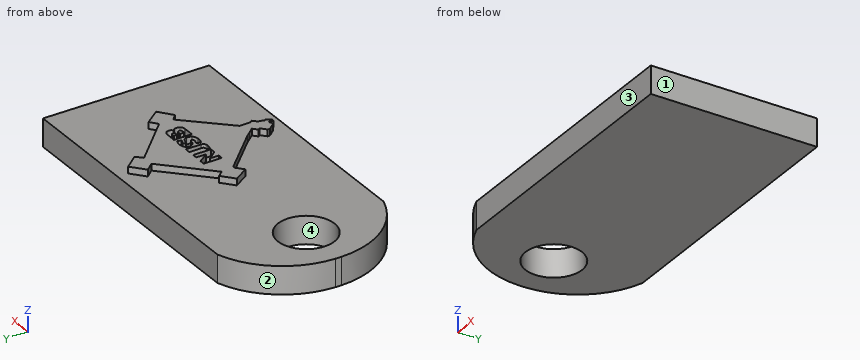
from build123d import *

# Parameters (mm, degrees)
F0_W     = 38.1
F0_H     = 19.05
F1_DEPTH = 3.175
F2_R     = 3.239621
F3_DEPTH = 3.176
F5_DEPTH = 0.762


with BuildPart() as f1:
    # F0 (on Top) → F1 (new body)
    with BuildSketch(Plane.XY):
        with Locations((-19.05, 9.525)):
            Rectangle(F0_W, F0_H)
    extrude(amount=F1_DEPTH)

    # F2 (on face) → F3 (cut, through all)
    with BuildSketch(Plane.XY.offset(3.175)):
        with BuildLine():
            ThreePointArc((-38.1, 9.877407), (-36.161286, 15.559844), (-31.275846, 19.05))
            Line((-31.275846, 19.05), (-38.1, 19.05))
            Line((-38.1, 19.05), (-38.1, 9.877407))
        make_face()
        with BuildLine():
            ThreePointArc((-31.275846, 0), (-36.161286, 3.490156), (-38.1, 9.172593))
            Line((-38.1, 9.172593), (-38.1, 0))
            Line((-38.1, 0), (-31.275846, 0))
        make_face()
        with Locations((-32.302372, 9.525)):
            Circle(F2_R)
    extrude(amount=-F3_DEPTH, mode=Mode.SUBTRACT)

    # F4 (on face) → F5 (join)
    with BuildSketch(Plane.XY.offset(3.175)):
        Polygon((-12.133155, 16.323839), (-13.419535, 17.867444), (-14.930828, 16.581235), (-14.155187, 15.669858), (-19.111004, 10.793301), (-19.653987, 11.431306), (-21.029584, 10.260583), (-19.947039, 8.606749), (-19.111004, 9.318269), (-18.885918, 9.318269), (-14.609277, 4.973212), (-14.512812, 5.356764), (-14.512812, 5.616316), (-14.239308, 6.20037), (-14.159105, 6.484506), (-12.678197, 6.066489), (-12.678197, 5.356764), (-12.937207, 5.101833), (-12.937207, 4.555195), (-12.549366, 4.555195), (-8.081773, 9.282008), (-7.436184, 8.671823), (-5.89522, 9.860801), (-7.199443, 11.551126), (-8.05396, 10.891797), (-12.808586, 15.648736), align=None)
        Polygon((-16.313503, 9.314163), (-16.86014, 9.346317), (-16.86014, 11.40425), (-16.281348, 11.40425), (-15.445312, 10.214509), (-15.445312, 11.372095), (-14.898674, 11.372095), (-14.898674, 9.314163), (-15.509622, 9.314163), (-16.313503, 10.310974), align=None, mode=Mode.SUBTRACT)
        with BuildLine():
            Line((-14.210255, 9.967692), (-14.223414, 11.372095))
            Line((-14.223414, 11.372095), (-13.580311, 11.372095))
            Line((-13.580311, 11.372095), (-13.580311, 9.642933))
            ThreePointArc((-13.580311, 9.642933), (-13.703139, 9.33071), (-14.005777, 9.185865))
            ThreePointArc((-14.005777, 9.185865), (-14.361345, 9.206839), (-14.703408, 9.306146))
            Line((-14.703408, 9.306146), (-14.595155, 9.691046))
            ThreePointArc((-14.595155, 9.691046), (-14.309597, 9.699827), (-14.210255, 9.967692))
        make_face(mode=Mode.SUBTRACT)
        with BuildLine():
            Line((-12.309813, 11.38701), (-11.792604, 11.230645))
            Line((-11.792604, 11.230645), (-11.919432, 10.779702))
            Line((-11.919432, 10.779702), (-12.419279, 10.920285))
            ThreePointArc((-12.419279, 10.920285), (-12.566064, 10.888649), (-12.622545, 10.74952))
            ThreePointArc((-12.622545, 10.74952), (-12.370625, 10.614414), (-12.093307, 10.545042))
            ThreePointArc((-12.093307, 10.545042), (-11.848866, 10.36705), (-11.732464, 10.087973))
            ThreePointArc((-11.732464, 10.087973), (-11.733256, 9.7951), (-11.840717, 9.522652))
            ThreePointArc((-11.840717, 9.522652), (-12.10655, 9.335291), (-12.419279, 9.246006))
            Line((-12.419279, 9.246006), (-12.827022, 9.246006))
            Line((-12.827022, 9.246006), (-13.272062, 9.390343))
            Line((-13.272062, 9.390343), (-13.113701, 9.878622))
            Line((-13.113701, 9.878622), (-12.726019, 9.752887))
            ThreePointArc((-12.726019, 9.752887), (-12.49708, 9.751795), (-12.309813, 9.883496))
            ThreePointArc((-12.309813, 9.883496), (-12.54216, 10.088347), (-12.851078, 10.111114))
            ThreePointArc((-12.851078, 10.111114), (-13.120867, 10.31145), (-13.28409, 10.605182))
            ThreePointArc((-13.28409, 10.605182), (-13.263213, 10.944513), (-13.079613, 11.230645))
            ThreePointArc((-13.079613, 11.230645), (-12.708492, 11.376665), (-12.309813, 11.38701))
        make_face(mode=Mode.SUBTRACT)
        with BuildLine():
            Line((-11.43176, 9.294118), (-11.43176, 11.350926))
            Line((-11.43176, 11.350926), (-10.087523, 11.330864))
            Line((-10.087523, 11.330864), (-9.940274, 11.266729))
            ThreePointArc((-9.940274, 11.266729), (-9.644752, 10.815674), (-9.940274, 10.36462))
            ThreePointArc((-9.940274, 10.36462), (-9.820796, 10.300702), (-9.711741, 10.220283))
            ThreePointArc((-9.711741, 10.220283), (-9.661743, 9.61308), (-10.180837, 9.294118))
            Line((-10.180837, 9.294118), (-11.43176, 9.294118))
        make_face(mode=Mode.SUBTRACT)
        with BuildLine():
            Line((-10.445168, 10.196227), (-10.770215, 10.208255))
            Line((-10.770215, 10.208255), (-10.770215, 9.751187))
            Line((-10.770215, 9.751187), (-10.445168, 9.746336))
            ThreePointArc((-10.445168, 9.746336), (-10.216841, 9.971281), (-10.445168, 10.196227))
        make_face()
        with BuildLine():
            Line((-10.770215, 10.929941), (-10.770215, 10.55707))
            Line((-10.770215, 10.55707), (-10.493567, 10.55707))
            ThreePointArc((-10.493567, 10.55707), (-10.307132, 10.743506), (-10.493567, 10.929941))
            Line((-10.493567, 10.929941), (-10.770215, 10.929941))
        make_face()
        Polygon((-12.549366, 3.912091), (-12.549366, 4.555195), (-12.937207, 4.555195), (-12.937207, 5.101833), (-12.678197, 5.356764), (-12.678197, 6.066489), (-14.159105, 6.484506), (-14.239308, 6.20037), (-14.512812, 5.616316), (-14.512812, 5.356764), (-14.609277, 4.973212), (-14.421192, 4.752211), (-14.170298, 4.457412), (-13.643861, 3.838849), (-14.170298, 3.390817), (-13.987954, 3.176562), (-14.609277, 2.647775), (-14.609277, 2.368642), (-14.346565, 2.059955), (-13.987954, 1.638587), (-13.643861, 1.638587), (-13.430775, 1.819937), (-13.430775, 1.24321), (-13.162293, 1.24321), (-12.872897, 1.819937), (-13.028217, 1.897875), (-12.827437, 2.298001), (-12.827437, 2.561572), (-12.326258, 3.0439), (-12.549366, 3.275728), align=None)
    extrude(amount=F5_DEPTH)


solid = f1.part
Can you work these out from the model? Positions are in its coordinate system, mm. Face numbers are marked on the shaded views. Give positions to 0.01 mm unless a question says otherwise; leave off trailing zeros. Write each loop counter-clockwise with the first axis right and the second up, starting at its lowest first coordinate (ties: lowest second). Pieces come first, ordered by that corner, then holes. Notation, with made-up numbers: M -10,-9.75 L 17,-9.75 A29 cw 17,17.25 Z; hole C -36.5,0 d6. An arc over 180 degrees is marked long. Answer in a Markdown table with one row per item. Add a question column.
Item 1: Imagine slicing it at C-C, the plane z = 2. Write out the boundary of the cut face in (x, y) (3 decimals).
Item 2: We'd pull the mould along X, two halves only. Please class the marked faces 1, 2, 3 and 4: released by +X, released by -X, zero draft, split by the parting line, or undercut.
Item 3: For pin 1 Ø1.2 at (x, y) = (-14, 10) entering from +Z, with a flat end and sliding along its axis, tell me the tip position at first contact or that it passes through.
Item 4: Imagine slicing it at D-D, the plane x = -18.5. Write out the boundary of the cut face in (y, z) (3 decimals), plus the area to 3 significant figures.
Item 5: Please list where these lines run through material, in increasing order: L1, parallel to Z at x = -29, y = 7 (3 decimals); L2, parallel to X at y = 9.5, z = 0.8; L3, parallel to Y at x = -31, z = 0.85.
Item 6: Imagine slicing it at B-B, the plane x = -32. Write out the boundary of the cut face in (y, z) (3 decimals), plus the area to 3 significant figures.
Item 7: Imagine slicing it at A-A, the plane y = 7.25. Write out the boundary of the cut face in (x, z) (3 decimals).
Evaluation:
| question | item | result |
|---|---|---|
| 1 | outline | M -38.1,9.173 A9.815 ccw -31.276,0 L 0,0 L 0,19.05 L -31.276,19.05 A9.815 ccw -38.1,9.877 Z; hole C -32.302,9.525 d6.479 |
| 2 | face 1 | released by +X |
| 2 | face 2 | released by -X |
| 2 | face 3 | zero draft |
| 2 | face 4 | undercut |
| 3 | pin 1 | stops at z = 3.94 |
| 4 | outline | M 0,0 L 19.05,0 L 19.05,3.175 L 11.395,3.175 L 11.395,3.937 L 8.926,3.937 L 8.926,3.175 L 0,3.175 Z |
| 4 | area | 62.4 mm² |
| 5 | L1 | z = 0 to 3.175 |
| 5 | L2 | x = -38.1 to -35.54, -29.06 to 0 |
| 5 | L3 | y = 0 to 6.56, 12.49 to 19.05 |
| 6 | outline | M 0.263,0 L 6.3,0 L 6.3,3.175 L 0.263,3.175 Z; M 12.75,0 L 18.787,0 L 18.787,3.175 L 12.75,3.175 Z |
| 6 | area | 38.3 mm² |
| 7 | outline | M -37.875,0 L -34.609,0 L -34.609,3.175 L -37.875,3.175 Z; M -29.996,0 L 0,0 L 0,3.175 L -10.002,3.175 L -10.002,3.937 L -16.85,3.937 L -16.85,3.175 L -29.996,3.175 Z |
